Verification items for the finished model (mm, model axes). Face numbers are marked on the shaded views. Coordinates: 2 decimals unless noted, no trailing zeros. Write each loop counter-clockwise with the first axis right and the second up, starting at its lowest first coordinate (ties: lowest second). Pieces come first, ordered by that corner, then holes. Notation, with made-up numbers: (-40, 60.25) - (-27, 60.25) arc R27 cw to (-27, 91.25) - close; hole circle Ø6 at (81.25, 10). An arc over 180 degrees is marked (long way). Answer as CSV lines item,"result". Start each with the question number.
```python
from build123d import *

# Parameters (mm, degrees)
SKETCH_1_W          = 30
SKETCH_1_H          = 30
SKETCH_1_W_2        = 26
SKETCH_1_H_2        = 26
EXTRUDE_1_DEPTH     = 350
SKETCH_2_R          = 1.75
CUT_EXTRUDE_1_DEPTH = 352.603469835
SKETCH_3_R          = 1.65
CUT_EXTRUDE_2_DEPTH = 352.603469835
SKETCH_4_R          = 2.1
CUT_EXTRUDE_3_DEPTH = 352.603469835
SKETCH_5_R          = 2.1
CUT_EXTRUDE_4_DEPTH = 352.603469835
SKETCH_6_R          = 2.5
CUT_EXTRUDE_5_DEPTH = 352.603469835


with BuildPart() as part:
    # 草图1 → 凸台-拉伸1 (new body)
    with BuildSketch(Plane(origin=(0, 0, 0), x_dir=(0, 0, -1), z_dir=(1, 0, 0))):
        Rectangle(SKETCH_1_W, SKETCH_1_H)
        Rectangle(SKETCH_1_W_2, SKETCH_1_H_2, mode=Mode.SUBTRACT)
    extrude(amount=EXTRUDE_1_DEPTH)

    # 草图2 → 切除-拉伸1 (cut, through all)
    with BuildSketch(Plane(origin=(0, 0, -15), x_dir=(-1, 0, 0), z_dir=(0, 0, -1))):
        with Locations((-307, 0)):
            Circle(SKETCH_2_R)
        with Locations((-287, 0)):
            Circle(SKETCH_2_R)
        with Locations((-267, 0)):
            Circle(SKETCH_2_R)
        with Locations((-247, 0)):
            Circle(SKETCH_2_R)
        with Locations((-227, 0)):
            Circle(SKETCH_2_R)
        with Locations((-207, 0)):
            Circle(SKETCH_2_R)
        with Locations((-187, 0)):
            Circle(SKETCH_2_R)
        with Locations((-167, 0)):
            Circle(SKETCH_2_R)
        with Locations((-147, 0)):
            Circle(SKETCH_2_R)
        with Locations((-127, 0)):
            Circle(SKETCH_2_R)
        with Locations((-107, 0)):
            Circle(SKETCH_2_R)
        with Locations((-87, 0)):
            Circle(SKETCH_2_R)
        with Locations((-67, 0)):
            Circle(SKETCH_2_R)
        with Locations((-47, 0)):
            Circle(SKETCH_2_R)
        with Locations((-27, 0)):
            Circle(SKETCH_2_R)
    extrude(amount=-CUT_EXTRUDE_1_DEPTH, mode=Mode.SUBTRACT)

    # 草图3 → 切除-拉伸2 (cut, through all)
    with BuildSketch(Plane.XY.offset(15)):
        with Locations((6, 7.724871585)):
            Circle(SKETCH_3_R)
        with Locations((6, -7.275128415)):
            Circle(SKETCH_3_R)
    extrude(amount=-CUT_EXTRUDE_2_DEPTH, mode=Mode.SUBTRACT)

    # 草图4 → 切除-拉伸3 (cut, through all)
    with BuildSketch(Plane(origin=(0, 15, 0), x_dir=(1, 0, 0), z_dir=(0, 1, 0))):
        with Locations(Location((326, 6, 0), (0, 0, 270))):
            Circle(SKETCH_4_R)
        with Locations(Location((326, -6, 0), (0, 0, 270))):
            Circle(SKETCH_4_R)
    extrude(amount=-CUT_EXTRUDE_3_DEPTH, mode=Mode.SUBTRACT)

    # 草图5 → 切除-拉伸4 (cut, through all)
    with BuildSketch(Plane.XZ.offset(15)):
        with Locations(Location((10.831487119, 6, 0), (0, 0, 270))):
            Circle(SKETCH_5_R)
        with Locations(Location((10.831487119, -6, 0), (0, 0, 270))):
            Circle(SKETCH_5_R)
    extrude(amount=-CUT_EXTRUDE_4_DEPTH, mode=Mode.SUBTRACT)

    # 草图6 → 切除-拉伸5 (cut, through all)
    with BuildSketch(Plane(origin=(0, 0, -15), x_dir=(-1, 0, 0), z_dir=(0, 0, -1))):
        with Locations((-331.15, 8.1)):
            Circle(SKETCH_6_R)
        with Locations((-300.95, 8.1)):
            Circle(SKETCH_6_R)
    extrude(amount=-CUT_EXTRUDE_5_DEPTH, mode=Mode.SUBTRACT)


solid = part.part
```
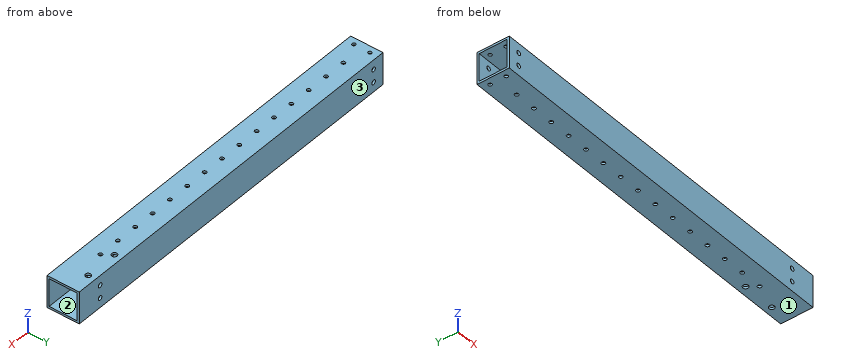
1. Draft check along Z on the marked faces 1, 2 and 3. Enter one of: pulls with the +Z half, pulls with the -Z half, needs draft (parallel to the pull), parting line crosses it, or undercut.
2. Depth check by flat-ended pin: P1, Ø2.5, axis at x = 10.83, z = 6, coming from the +Y side; P2, Ø4.5, axis at x = 167, y = 0, coming from the -Z side. Enter the tip coordinate at first touch or a pass-through.
3. Scan lines: line 1 along Y through (x, z) = (6, -14.45); line 2 along Z through (x, y) = (326, -13.45); line 3 along Z through (x, y) = (40, 0). Record each from-to range of solid material in increasing order. Write a range as from..to.
4. Cross-section at A-A (x = 254). Record the cut outline in (y, z), and give its area (3 significant figures).
Completed:
1,face 1,"pulls with the -Z half"
1,face 2,"undercut"
1,face 3,"needs draft"
2,P1,"passes through"
2,P2,"stops at z = -15"
3,line 1,"y = -15..-8.93, -5.63..6.07, 9.37..15"
3,line 2,"z = -15..-8.1, -3.9..3.9, 8.1..15"
3,line 3,"z = -15..-13, 13..15"
4,outline,"(-15, -15) - (15, -15) - (15, 15) - (-15, 15) - close; hole (-13, -13) - (13, -13) - (13, 13) - (-13, 13) - close"
4,area,"224 mm2"
